Can you work these out from the model? Positions are in its coordinate system, mm. Face numbers are marked on the shaded views. A direction names the side the tool comes from. Give positions to 0.01 mm unless a question says otherwise; leave off trailing zeros. Order: outer loops, then holes, each group sorted by start corner. A loop starts at its lowest first (then second) coordinate and runs counter-clockwise, first axis right, second up. Notation, with made-up numbers: M -7.75,-15 L 0.25,-15 A12 ccw 0.25,-11 Z; hole C 23,22.25 d5. An arc over 180 degrees is marked long. One line per question, with ' | ' between items. Start each with the question number.
1) Please list where these lines run through material, in increasing order: line 1 along X through (y, z) = (3.25, 0); line 2 along Z through (x, y) = (-11, 36); line 3 along Z through (x, y) = (8.5, 27.5). Write a range as [from, to].
2) I'm going to push flat-ended pins straight in: pin 1 Ø1 at (x, z) = (9.5, -18) entering from -Y; pin 2 Ø3 at (x, y) = (3, 6) entering from +Z; pin 3 Ø9.5 at (x, z) = (0, -27) entering from +Y; pin 4 Ø12 at (y, z) = (18.5, -24) entering from +X. Where does each tip first touch, or does it pass through?
3) If we section it at A-A, the plane z = 0: Please give me the cut outline in (x, y), plus the area to 3 significant figures.
4) If we section it at C-C, the plane y = 2: Please give me the cut outline in (x, z), plus the area to 3 significant figures.
5) If we section it at D-D, the plane z = -27: Please give me the cut outline in (x, y).
6) If we section it at B-B, the plane x = 0: Please give me the cut outline in (y, z).
7) For the marked faces 4 and 5, which set-ups out of +Z, -Z, +X, -X, +Y, -Y let a thin tool reach every point of the face, with its end or its side?
8) Thinking about a two-plate mould opening in X: for the marked faces 1, 2 and 3, which applies, +X half, -X half, draft (parallel to the pull), parting line (faces both ways), or undercut?
```python
from build123d import *

# Parameters (mm, degrees)
SKETCH_1_R      = 3
EXTRUDE_1_DEPTH = 6
SKETCH_2_R      = 22.5
EXTRUDE_2_DEPTH = 33
CHAMFER_1_SIZE  = 1


with BuildPart() as part:
    # 草图1 → 凸台-拉伸1 (new body)
    with BuildSketch(Plane(origin=(0, 0, 0), x_dir=(1, 0, 0), z_dir=(0, 1, 0))):
        with BuildLine():
            Line((11.489125293, 32), (-11.489125293, 32))
            ThreePointArc((-11.489125293, 32), (0, -34), (11.489125293, 32))
        make_face()
        with Locations(Location((0, 27, 0), (0, 0, 270))):
            Circle(SKETCH_1_R, mode=Mode.SUBTRACT)
        with Locations(Location((27, 0, 0), (0, 0, 270))):
            Circle(SKETCH_1_R, mode=Mode.SUBTRACT)
        with Locations(Location((0, -27, 0), (0, 0, 270))):
            Circle(SKETCH_1_R, mode=Mode.SUBTRACT)
        with Locations(Location((-27, 0, 0), (0, 0, 270))):
            Circle(SKETCH_1_R, mode=Mode.SUBTRACT)
    extrude(amount=EXTRUDE_1_DEPTH)

    # 草图2 → 凸台-拉伸2 (add)
    with BuildSketch(Plane(origin=(0, 6, 0), x_dir=(1, 0, 0), z_dir=(0, 1, 0))):
        with Locations(Location((0, 0, 0), (0, 0, 270))):
            Circle(SKETCH_2_R)
    extrude(amount=EXTRUDE_2_DEPTH)

    # 草图3 → 切除-旋转1 (revolve, cut)
    with BuildSketch(Plane.XY):
        Polygon((0, 39), (16, 39), (16, 35), (18.5, 35), (18.5, 0), (0, 0), align=None)
    revolve(axis=Axis((0, 0, 0), (0, 1, 0)), mode=Mode.SUBTRACT)

    # 倒角1
    chamfer_1_edges = [part.edges().sort_by_distance(p)[0] for p in [
        (0, 39, -22.5),
        (-18.5, 0, 0),
    ]]
    chamfer(chamfer_1_edges, length=CHAMFER_1_SIZE)


solid = part.part
```
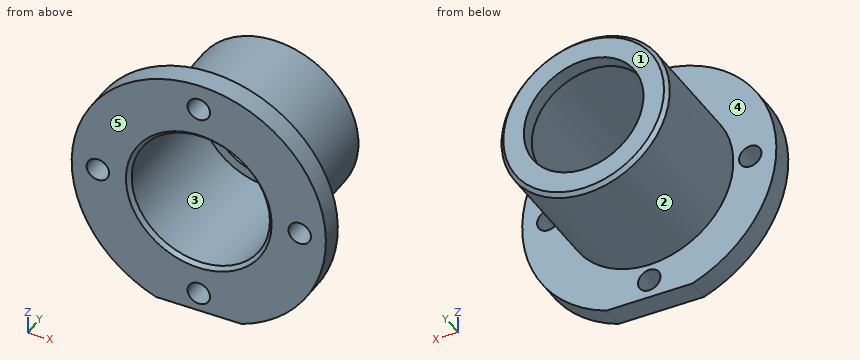
Results found:
1) line 1: x = [-34, -30], [-24, -18.5], [18.5, 24], [30, 34] | line 2: z = [-19.63, -11.62], [11.62, 19.63] | line 3: z = [-20.83, -16.43], [16.43, 20.83]
2) pin 1: stops at y = 0 | pin 2: stops at z = 33.97 | pin 3: stops at y = 38.25 | pin 4: stops at x = 13.5
3) outline: M -34,0 L -30,0 L -30,6 L -34,6 Z; M -24,0 L -19.5,0 L -18.5,1 L -18.5,35 L -16,35 L -16,39 L -21.5,39 L -22.5,38 L -22.5,6 L -24,6 Z; M 16,35 L 18.5,35 L 18.5,1 L 19.5,0 L 24,0 L 24,6 L 22.5,6 L 22.5,38 L 21.5,39 L 16,39 Z; M 30,0 L 34,0 L 34,6 L 30,6 Z | area: 396 mm²
4) outline: M -11.49,-32 L 11.49,-32 A34 ccw long Z; hole C -27,0 d6; hole C 0,0 d37; hole C 0,-27 d6; hole C 0,27 d6; hole C 27,0 d6 | area: 2,410 mm²
5) outline: M -20.66,0 L -3,0 L -3,6 L -20.66,6 Z; M 3,0 L 20.66,0 L 20.66,6 L 3,6 Z
6) outline: M 0,-32 L 6,-32 L 6,-30 L 0,-30 Z; M 0,-24 L 6,-24 L 6,-22.5 L 38,-22.5 L 39,-21.5 L 39,-16 L 35,-16 L 35,-18.5 L 1,-18.5 L 0,-19.5 Z; M 0,19.5 L 1,18.5 L 35,18.5 L 35,16 L 39,16 L 39,21.5 L 38,22.5 L 6,22.5 L 6,24 L 0,24 Z; M 0,30 L 6,30 L 6,34 L 0,34 Z
7) face 4: +Y | face 5: +Z, -Z, +X, -X, -Y
8) face 1: draft | face 2: parting line | face 3: undercut
